Design review of the part shown in the three views and the two pictorial views. Dimensions are in mm from the part's minimum x, y and z. Coordinates: 2 decimals unless noted, no trailing zeros. Write each loop counter-clockwise with the first axis right and the second up, starting at its lowest first coordinate (ties: lowest second). Pieces come first, ordered by that corner, then holes. Notation, with made-up numbers: (-1, -38) -> (37, -38) arc R21 ccw to (37, -13) -> close; hole circle Ø11 at (33, -16.75). An arc over 180 degrees is marked (long way). Answer in a Markdown table with one row per item. Add a question column.
Item 1: Take a section at B-B, the plane z = 73. Write out the cut boundary in (x, y), and give its area (3 significant figures).
Item 2: To check wall thickness, follow line 1 (Z direction, x = 214, y = 0.7); line 2 (X direction, y = 1.05, z = 91); line 3 (X direction, y = 0.65, z = 11). State the ranges of each line that lie inside material, in increasing order.
Item 3: Take a section at A-A, the plane x = 77. Write out the cut boundary in (y, z), and give its area (3 significant figures).
Item 4: Clearance check with a flat-ended pin moving along its axis: P1, Ø4, axis at x = 10, z = 73, coming from the +Y side. State where the tip first meets the part, or that it passes through.
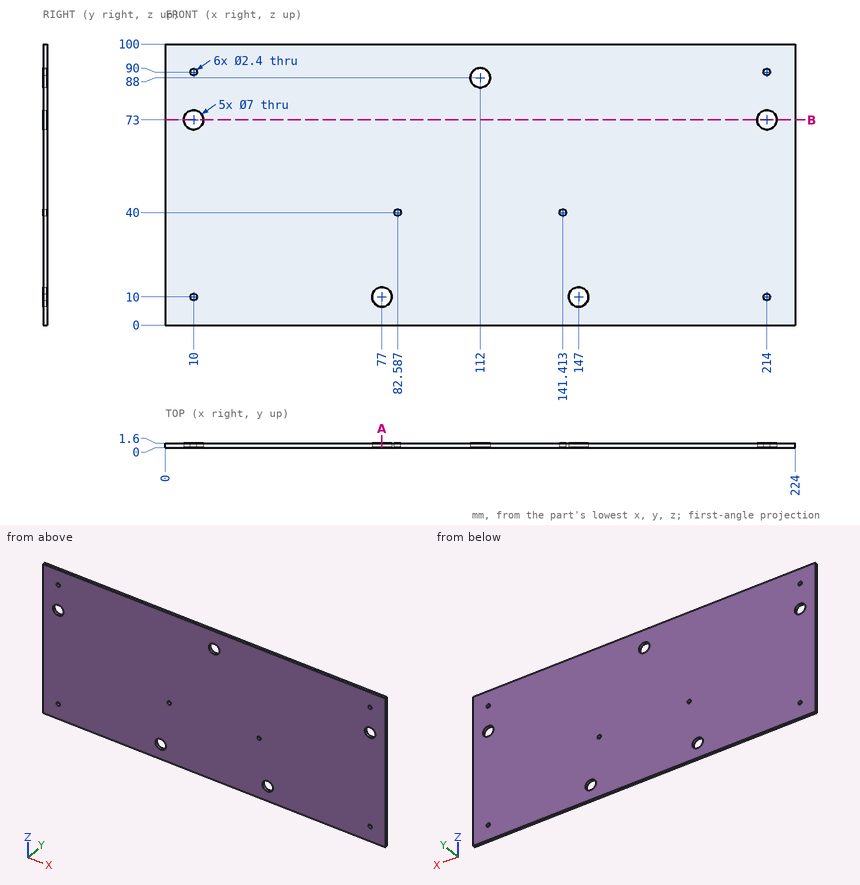
Answers:
| question | item | result |
|---|---|---|
| 1 | outline | (0, 0) -> (6.5, 0) -> (6.5, 1.6) -> (0, 1.6) -> close; (13.5, 0) -> (210.5, 0) -> (210.5, 1.6) -> (13.5, 1.6) -> close; (217.5, 0) -> (224, 0) -> (224, 1.6) -> (217.5, 1.6) -> close |
| 1 | area | 336 mm^2 |
| 2 | line 1 | z = 0 to 8.8, 11.2 to 69.5, 76.5 to 88.8, 91.2 to 100 |
| 2 | line 2 | x = 0 to 9.34, 10.66 to 110.2, 113.8 to 213.34, 214.66 to 224 |
| 2 | line 3 | x = 0 to 9.34, 10.66 to 73.65, 80.35 to 143.65, 150.35 to 213.34, 214.66 to 224 |
| 3 | outline | (0, 0) -> (1.6, 0) -> (1.6, 6.5) -> (0, 6.5) -> close; (0, 13.5) -> (1.6, 13.5) -> (1.6, 100) -> (0, 100) -> close |
| 3 | area | 149 mm^2 |
| 4 | P1 | passes through |
